Design review of the part built by this model. Coordinates are the model's own, in mm. A direction names the side the tool comes from. Round coordinates to 2 decimals unless told otherwise and drop trailing zeros. Write each loop counter-clockwise with the first axis right and the second up, starting at its lowest first coordinate (ties: lowest second). Pieces come first, ordered by that corner, then holes. Notation, with made-up numbers: (-4, 14) - (34, 14) arc R18 ccw to (34, 27) - close; hole circle Ø9 at (62, -15). An arc over 180 degrees is marked (long way). Use one line per item in the form item = value.
```python
from build123d import *

# Parameters (mm, degrees)
F0_W      = 42
F0_H      = 23
F1_DEPTH  = 5
F3_ANGLE  = 90
F8_R      = 2.05
F9_DEPTH  = 5
F10_DEPTH = 3


# Not quite as in the source:
# - a feature names something its author has since deleted; it is built from what else it names


with BuildPart() as f1:
    # F0 (on Top) → F1 (new body)
    with BuildSketch(Plane.XY):
        Rectangle(F0_W, F0_H)
        with BuildLine():
            ThreePointArc((-16, -9.55), (-18.05, -7.5), (-16, -5.45))
            Line((-16, -5.45), (16, -5.45))
            ThreePointArc((16, -5.45), (18.05, -7.5), (16, -9.55))
            Line((16, -9.55), (-16, -9.55))
        make_face(mode=Mode.SUBTRACT)
        with BuildLine():
            Line((0, -1.55), (-16, -1.55))
            ThreePointArc((-16, -1.55), (-18.05, 0.5), (-16, 2.55))
            Line((-16, 2.55), (0, 2.55))
            Line((0, 2.55), (16, 2.55))
            ThreePointArc((16, 2.55), (18.05, 0.5), (16, -1.55))
            Line((16, -1.55), (0, -1.55))
        make_face(mode=Mode.SUBTRACT)
        with BuildLine():
            Line((16, 6.45), (-16, 6.45))
            ThreePointArc((-16, 6.45), (-18.05, 8.5), (-16, 10.55))
            Line((-16, 10.55), (16, 10.55))
            ThreePointArc((16, 10.55), (18.05, 8.5), (16, 6.45))
        make_face(mode=Mode.SUBTRACT)
    extrude(amount=F1_DEPTH)


with BuildPart() as f3_1:
    # F3: copy of F1
    add(f1.part.rotate(Axis((-21, 0, 2.5), (0, -1, 0)), F3_ANGLE))


with BuildPart() as f3_1_1:
    # F4: moved
    add(f3_1.part.moved(Location((0, 0, 14))))


with BuildPart() as f3_1_2:
    # F5: moved
    add(f3_1_1.part.moved(Location((-14, 0, 0))))


with BuildPart() as f1_1:
    add(f1.part)

    add(f3_1_2.part)  # F9 merges F3_1
    # F8 (on 3pt) → F9 (join)
    with BuildSketch(Plane.XZ.offset(11.5)):
        Polygon((-37.5, 16.5), (-21, 0), (21, 0), (21, 5), (14.4509618943, 11.5490381057), (13.5, 11), (10.0358983849, 13), (10.0358983849, 15.9641016151), (2.4509618943, 23.5490381057), (1.5, 23), (-1.9641016151, 25), (-1.9641016151, 27.9641016151), (-9.5490381057, 35.5490381057), (-10.5, 35), (-13.9641016151, 37), (-13.9641016151, 39.9641016151), (-21.5490381057, 47.5490381057), (-22.5, 47), (-25.9641016151, 49), (-25.9641016151, 51.9641016151), (-32.5, 58.5), (-37.5, 58.5), align=None)
        Polygon((-25.9641016151, 17), (-22.5, 19), (-19.0358983849, 17), (-19.0358983849, 13), (-22.5, 11), (-25.9641016151, 13), align=None, mode=Mode.SUBTRACT)
        Polygon((-13.9641016151, 13), (-13.9641016151, 17), (-10.5, 19), (-7.0358983849, 17), (-7.0358983849, 13), (-10.5, 11), align=None, mode=Mode.SUBTRACT)
        Polygon((-25.9641016151, 25), (-25.9641016151, 29), (-22.5, 31), (-19.0358983849, 29), (-19.0358983849, 25), (-22.5, 23), align=None, mode=Mode.SUBTRACT)
        Polygon((-13.9641016151, 25), (-13.9641016151, 29), (-10.5, 31), (-7.0358983849, 29), (-7.0358983849, 25), (-10.5, 23), align=None, mode=Mode.SUBTRACT)
        Polygon((-1.9641016151, 13), (-1.9641016151, 17), (1.5, 19), (4.9641016151, 17), (4.9641016151, 13), (1.5, 11), align=None, mode=Mode.SUBTRACT)
        Polygon((-25.9641016151, 37), (-25.9641016151, 41), (-22.5, 43), (-19.0358983849, 41), (-19.0358983849, 37), (-22.5, 35), align=None, mode=Mode.SUBTRACT)
        with BuildLine():
            Line((13.5, 11), (14.4509618943, 11.5490381057))
            Line((14.4509618943, 11.5490381057), (12.9839959128, 13.0160040872))
            ThreePointArc((12.9839959128, 13.0160040872), (12.0504310986, 13.5504310986), (11.5160040872, 14.4839959128))
            Line((11.5160040872, 14.4839959128), (10.0358983849, 15.9641016151))
            Line((10.0358983849, 15.9641016151), (10.0358983849, 13))
            Line((10.0358983849, 13), (13.5, 11))
        make_face()
        with BuildLine():
            Line((-24.4839959128, 50.4839959128), (-25.9641016151, 51.9641016151))
            Line((-25.9641016151, 51.9641016151), (-25.9641016151, 49))
            Line((-25.9641016151, 49), (-22.5, 47))
            Line((-22.5, 47), (-21.5490381057, 47.5490381057))
            Line((-21.5490381057, 47.5490381057), (-23.0160040872, 49.0160040872))
            ThreePointArc((-23.0160040872, 49.0160040872), (-23.9495689014, 49.5504310986), (-24.4839959128, 50.4839959128))
        make_face()
        with BuildLine():
            ThreePointArc((11.5160040872, 14.4839959128), (12.0504310986, 13.5504310986), (12.9839959128, 13.0160040872))
            Line((12.9839959128, 13.0160040872), (11.5160040872, 14.4839959128))
        make_face()
        with BuildLine():
            Line((-23.0160040872, 49.0160040872), (-24.4839959128, 50.4839959128))
            ThreePointArc((-24.4839959128, 50.4839959128), (-23.9495689014, 49.5504310986), (-23.0160040872, 49.0160040872))
        make_face()
        with BuildLine():
            Line((1.5, 23), (2.4509618943, 23.5490381057))
            Line((2.4509618943, 23.5490381057), (0.9839959128, 25.0160040872))
            ThreePointArc((0.9839959128, 25.0160040872), (0.0504310986, 25.5504310986), (-0.4839959128, 26.4839959128))
            Line((-0.4839959128, 26.4839959128), (-1.9641016151, 27.9641016151))
            Line((-1.9641016151, 27.9641016151), (-1.9641016151, 25))
            Line((-1.9641016151, 25), (1.5, 23))
        make_face()
        with BuildLine():
            Line((-12.4839959128, 38.4839959128), (-13.9641016151, 39.9641016151))
            Line((-13.9641016151, 39.9641016151), (-13.9641016151, 37))
            Line((-13.9641016151, 37), (-10.5, 35))
            Line((-10.5, 35), (-9.5490381057, 35.5490381057))
            Line((-9.5490381057, 35.5490381057), (-11.0160040872, 37.0160040872))
            ThreePointArc((-11.0160040872, 37.0160040872), (-11.9495689014, 37.5504310986), (-12.4839959128, 38.4839959128))
        make_face()
        with BuildLine():
            ThreePointArc((-0.4839959128, 26.4839959128), (0.0504310986, 25.5504310986), (0.9839959128, 25.0160040872))
            Line((0.9839959128, 25.0160040872), (-0.4839959128, 26.4839959128))
        make_face()
        with BuildLine():
            Line((-11.0160040872, 37.0160040872), (-12.4839959128, 38.4839959128))
            ThreePointArc((-12.4839959128, 38.4839959128), (-11.9495689014, 37.5504310986), (-11.0160040872, 37.0160040872))
        make_face()
        Polygon((-10.5, 31), (-13.9641016151, 29), (-13.9641016151, 25), (-10.5, 23), (-7.0358983849, 25), (-7.0358983849, 29), align=None)
        with Locations((-10.5, 27)):
            Circle(F8_R, mode=Mode.SUBTRACT)
        Polygon((-22.5, 31), (-25.9641016151, 29), (-25.9641016151, 25), (-22.5, 23), (-19.0358983849, 25), (-19.0358983849, 29), align=None)
        with Locations((-22.5, 27)):
            Circle(F8_R, mode=Mode.SUBTRACT)
        Polygon((-22.5, 43), (-25.9641016151, 41), (-25.9641016151, 37), (-22.5, 35), (-19.0358983849, 37), (-19.0358983849, 41), align=None)
        with Locations((-22.5, 39)):
            Circle(F8_R, mode=Mode.SUBTRACT)
        Polygon((-10.5, 19), (-13.9641016151, 17), (-13.9641016151, 13), (-10.5, 11), (-7.0358983849, 13), (-7.0358983849, 17), align=None)
        with Locations((-10.5, 15)):
            Circle(F8_R, mode=Mode.SUBTRACT)
        Polygon((1.5, 19), (-1.9641016151, 17), (-1.9641016151, 13), (1.5, 11), (4.9641016151, 13), (4.9641016151, 17), align=None)
        with Locations((1.5, 15)):
            Circle(F8_R, mode=Mode.SUBTRACT)
        Polygon((-19.0358983849, 17), (-22.5, 19), (-25.9641016151, 17), (-25.9641016151, 13), (-22.5, 11), (-19.0358983849, 13), align=None)
        with Locations((-22.5, 15)):
            Circle(F8_R, mode=Mode.SUBTRACT)
    extrude(amount=F9_DEPTH)

    # F8 (on 3pt) → F10 (cut)
    with BuildSketch(Plane.XZ.offset(11.5)):
        Polygon((-10.5, 31), (-13.9641016151, 29), (-13.9641016151, 25), (-10.5, 23), (-7.0358983849, 25), (-7.0358983849, 29), align=None)
        with Locations((-10.5, 27)):
            Circle(F8_R, mode=Mode.SUBTRACT)
        Polygon((-22.5, 31), (-25.9641016151, 29), (-25.9641016151, 25), (-22.5, 23), (-19.0358983849, 25), (-19.0358983849, 29), align=None)
        with Locations((-22.5, 27)):
            Circle(F8_R, mode=Mode.SUBTRACT)
        Polygon((-22.5, 43), (-25.9641016151, 41), (-25.9641016151, 37), (-22.5, 35), (-19.0358983849, 37), (-19.0358983849, 41), align=None)
        with Locations((-22.5, 39)):
            Circle(F8_R, mode=Mode.SUBTRACT)
        Polygon((-10.5, 19), (-13.9641016151, 17), (-13.9641016151, 13), (-10.5, 11), (-7.0358983849, 13), (-7.0358983849, 17), align=None)
        with Locations((-10.5, 15)):
            Circle(F8_R, mode=Mode.SUBTRACT)
        Polygon((1.5, 19), (-1.9641016151, 17), (-1.9641016151, 13), (1.5, 11), (4.9641016151, 13), (4.9641016151, 17), align=None)
        with Locations((1.5, 15)):
            Circle(F8_R, mode=Mode.SUBTRACT)
        with BuildLine():
            Line((0.9839959128, 25.0160040872), (2.4509618943, 23.5490381057))
            Line((2.4509618943, 23.5490381057), (4.9641016151, 25))
            Line((4.9641016151, 25), (4.9641016151, 29))
            Line((4.9641016151, 29), (1.5, 31))
            Line((1.5, 31), (-1.9641016151, 29))
            Line((-1.9641016151, 29), (-1.9641016151, 27.9641016151))
            Line((-1.9641016151, 27.9641016151), (-0.4839959128, 26.4839959128))
            ThreePointArc((-0.4839959128, 26.4839959128), (1.2398958105, 29.0334320275), (3.55, 27))
            ThreePointArc((3.55, 27), (2.7539321396, 25.3782249881), (0.9839959128, 25.0160040872))
        make_face()
        with BuildLine():
            Line((12.9839959128, 13.0160040872), (14.4509618943, 11.5490381057))
            Line((14.4509618943, 11.5490381057), (16.9641016151, 13))
            Line((16.9641016151, 13), (16.9641016151, 17))
            Line((16.9641016151, 17), (13.5, 19))
            Line((13.5, 19), (10.0358983849, 17))
            Line((10.0358983849, 17), (10.0358983849, 15.9641016151))
            Line((10.0358983849, 15.9641016151), (11.5160040872, 14.4839959128))
            ThreePointArc((11.5160040872, 14.4839959128), (13.2398958105, 17.0334320275), (15.55, 15))
            ThreePointArc((15.55, 15), (14.7539321396, 13.3782249881), (12.9839959128, 13.0160040872))
        make_face()
        Polygon((-19.0358983849, 17), (-22.5, 19), (-25.9641016151, 17), (-25.9641016151, 13), (-22.5, 11), (-19.0358983849, 13), align=None)
        with Locations((-22.5, 15)):
            Circle(F8_R, mode=Mode.SUBTRACT)
    extrude(amount=F10_DEPTH, mode=Mode.SUBTRACT)


solid = f1_1.part
```
Q1. Machinability: for faces 4 (the cylindrical face through (-34.96, -7.45, 55.55)), 5 (the flat face through (-24, -14.5, 25)), 6 (the flat face through (-32.5, -2, 37)), 7 (the cylindrical face through (-18.05, -7.55, 2.46)), which of the approach directions +Z, -Z, +X, -X, +Y, -Y give a long, thin tool a straight path to every point of the face, cutting with its end or side? Answer none if there is none.
Calculated:
face_4 = +X, -X
face_5 = +Y
face_6 = +Z, -Z, +X, +Y
face_7 = +Z, -Z
Q2. For P1, Ø12, axis at y = 1.5, z = 49, coming from the +X side; P2, Ø0.9, axis at y = -12.5, z = 15, coming from the -X side; P3, Ø2.5, axis at y = -12.5, z = 14, coming from the +X side, all flat-tipped, find the tip position at first contact; note any pin that passes through.
Calculated:
P1 = -32.5
P2 = -36.45
P3 = 13.25
Q3. To check wall thickness, follow line 1 along Z through (x, y) = (-22.5, -15.9); line 2 along Y through (x, z) = (8.5, 16); line 3 along Z through (x, y) = (-18, -3.5). State the ranges of each line that lie inside material, in increasing order. Write a range as from..to.
Calculated:
line_1 = 1.5..12.95, 17.05..24.95, 29.05..36.95, 41.05..48.5
line_2 = -16.5..-11.5
line_3 = 0..5
Q4. We need section C-C on z = 51. Write out the cut boundary in (x, y).
Calculated:
outline = (-37.5, -16.5) - (-25, -16.5) - (-25, -11.5) - (-32.5, -11.5) - (-32.5, -9.55) - (-37.5, -9.55) - close; (-37.5, -5.45) - (-32.5, -5.45) - (-32.5, -1.55) - (-37.5, -1.55) - close; (-37.5, 2.55) - (-32.5, 2.55) - (-32.5, 6.45) - (-37.5, 6.45) - close; (-37.5, 10.55) - (-32.5, 10.55) - (-32.5, 11.5) - (-37.5, 11.5) - close
Q5. We need section B-B on z = 39. Write out the cut boundary in (x, y).
Calculated:
outline = (-37.5, -16.5) - (-24.55, -16.5) - (-24.55, -14.5) - (-25.96, -14.5) - (-25.96, -11.5) - (-32.5, -11.5) - (-32.5, -9.55) - (-37.5, -9.55) - close; (-37.5, -5.45) - (-32.5, -5.45) - (-32.5, -1.55) - (-37.5, -1.55) - close; (-37.5, 2.55) - (-32.5, 2.55) - (-32.5, 6.45) - (-37.5, 6.45) - close; (-37.5, 10.55) - (-32.5, 10.55) - (-32.5, 11.5) - (-37.5, 11.5) - close; (-20.45, -16.5) - (-13, -16.5) - (-13, -11.5) - (-19.04, -11.5) - (-19.04, -14.5) - (-20.45, -14.5) - close
Q6. We need section D-D on y = 0.5. Write out the cut boundary in (x, z), then the cut area to 3 significant figures.
Calculated:
outline = (-37.5, 16.5) - (-32.5, 16.5) - (-32.5, 19.45) - (-37.5, 19.45) - close; (-37.5, 55.55) - (-32.5, 55.55) - (-32.5, 58.5) - (-37.5, 58.5) - close; (-21, 0) - (-18.05, 0) - (-18.05, 5) - (-21, 5) - close; (18.05, 0) - (21, 0) - (21, 5) - (18.05, 5) - close
area = 59.0 mm2
Q7. Draft analysis for pull direction Y (two halves, no side actions). For faces 1 (the flat face through (-24, -14.5, 13)), 2 (the flat face through (-35, 6.45, 38)), 3 (the flat face through (0, -2, 5)), state which applies: released by +Y, released by -Y, zero draft, split by the parting line, or undercut.
Calculated:
face_1 = released by +Y
face_2 = undercut
face_3 = zero draft
Q8. We need section A-A on x = 10. Write out the cut boundary in (y, z), then the cut area to 4 significant figures.
Calculated:
outline = (-16.5, 0) - (-9.55, 0) - (-9.55, 5) - (-11.5, 5) - (-11.5, 16) - (-16.5, 16) - close; (-5.45, 0) - (-1.55, 0) - (-1.55, 5) - (-5.45, 5) - close; (2.55, 0) - (6.45, 0) - (6.45, 5) - (2.55, 5) - close; (10.55, 0) - (11.5, 0) - (11.5, 5) - (10.55, 5) - close
area = 133.5 mm2
